```python
from build123d import *

# Parameters (mm, degrees)
SKETCH_2_R      = 3.5
EXTRUDE_3_DEPTH = 500


with BuildPart() as part:
    # Эскиз2 → Бобышка-Вытянуть3 (new body)
    with BuildSketch(Plane.XY):
        with BuildLine():
            Line((-4.25, 20.8), (4.25, 20.8))
            Line((4.25, 20.8), (8.25, 24.8))
            Line((8.25, 24.8), (8.25, 26.8))
            Line((8.25, 26.8), (4.1, 26.8))
            Line((4.1, 26.8), (4.1, 29))
            Line((4.1, 29), (9.55, 29))
            ThreePointArc((9.55, 29), (9.903553391, 29.146446609), (10.05, 29.5))
            Line((10.05, 29.5), (10.05, 30))
            Line((10.05, 30), (27.5, 30))
            ThreePointArc((27.5, 30), (29.267766953, 29.267766953), (30, 27.5))
            Line((30, 27.5), (30, 22.55))
            Line((30, 22.55), (29, 22.55))
            Line((29, 22.55), (29, 19.1))
            Line((29, 19.1), (26.8, 19.1))
            Line((26.8, 19.1), (26.8, 23.25))
            Line((26.8, 23.25), (24.8, 23.25))
            Line((24.8, 23.25), (20.8, 19.25))
            Line((20.8, 19.25), (20.8, 10.75))
            Line((20.8, 10.75), (24.8, 6.75))
            Line((24.8, 6.75), (26.8, 6.75))
            Line((26.8, 6.75), (26.8, 10.9))
            Line((26.8, 10.9), (29, 10.9))
            Line((29, 10.9), (29, 0))
            Line((29, 0), (25.8, 0))
            Line((25.8, 0), (25.8, 4.05))
            Line((25.8, 4.05), (23.398780669, 4.05))
            Line((23.398780669, 4.05), (19.248780669, 8.2))
            Line((19.248780669, 8.2), (15, 8.2))
            ThreePointArc((15, 8.2), (10.191673888, 10.191673888), (8.2, 15))
            ThreePointArc((8.2, 15), (7.965685425, 15.565685425), (7.4, 15.8))
            Line((7.4, 15.8), (-7.4, 15.8))
            ThreePointArc((-7.4, 15.8), (-7.965685425, 15.565685425), (-8.2, 15))
            ThreePointArc((-8.2, 15), (-10.191673888, 10.191673888), (-15, 8.2))
            Line((-15, 8.2), (-19.248780669, 8.2))
            Line((-19.248780669, 8.2), (-23.398780669, 4.05))
            Line((-23.398780669, 4.05), (-25.8, 4.05))
            Line((-25.8, 4.05), (-25.8, 0))
            Line((-25.8, 0), (-29, 0))
            Line((-29, 0), (-29, 10.9))
            Line((-29, 10.9), (-26.8, 10.9))
            Line((-26.8, 10.9), (-26.8, 6.75))
            Line((-26.8, 6.75), (-24.8, 6.75))
            Line((-24.8, 6.75), (-20.8, 10.75))
            Line((-20.8, 10.75), (-20.8, 19.25))
            Line((-20.8, 19.25), (-24.8, 23.25))
            Line((-24.8, 23.25), (-26.8, 23.25))
            Line((-26.8, 23.25), (-26.8, 19.1))
            Line((-26.8, 19.1), (-29, 19.1))
            Line((-29, 19.1), (-29, 22.55))
            Line((-29, 22.55), (-30, 22.55))
            Line((-30, 22.55), (-30, 27.5))
            ThreePointArc((-30, 27.5), (-29.267766953, 29.267766953), (-27.5, 30))
            Line((-27.5, 30), (-10.05, 30))
            Line((-10.05, 30), (-10.05, 29.5))
            ThreePointArc((-10.05, 29.5), (-9.903553391, 29.146446609), (-9.55, 29))
            Line((-9.55, 29), (-4.1, 29))
            Line((-4.1, 29), (-4.1, 26.8))
            Line((-4.1, 26.8), (-8.25, 26.8))
            Line((-8.25, 26.8), (-8.25, 24.8))
            Line((-8.25, 24.8), (-4.25, 20.8))
        make_face()
        with Locations((15, 15)):
            Circle(SKETCH_2_R, mode=Mode.SUBTRACT)
        with Locations(Location((-15, 15, 0), (0, 0, 180))):
            Circle(SKETCH_2_R, mode=Mode.SUBTRACT)
        with BuildLine():
            Line((14, 26.75), (19, 26.75))
            ThreePointArc((19, 26.75), (21.5, 24.25), (19, 21.75))
            Line((19, 21.75), (14, 21.75))
            ThreePointArc((14, 21.75), (11.5, 24.25), (14, 26.75))
        make_face(mode=Mode.SUBTRACT)
        with BuildLine():
            Line((-14, 21.75), (-19, 21.75))
            ThreePointArc((-19, 21.75), (-21.5, 24.25), (-19, 26.75))
            Line((-19, 26.75), (-14, 26.75))
            ThreePointArc((-14, 26.75), (-11.5, 24.25), (-14, 21.75))
        make_face(mode=Mode.SUBTRACT)
    extrude_3 = extrude(amount=EXTRUDE_3_DEPTH)

    # Зеркальное отражение13: Бобышка-Вытянуть3 across plane
    add(extrude_3.mirror(Plane(origin=(25.8, 0, 500), x_dir=(0, 0, 1), z_dir=(0, 1, 0))))


solid = part.part
```
The listing builds one solid part. Answer for the finished solid, in the listing's coordinates (mm). A direction names the side the tool comes from. Round coordinates to 2 decimals unless told otherwise and drop trailing zeros. Use one line per item in the form item = value. Start each with the question number.
1. A tool of negligible diameter and unlimited length cuts with its end or side. For faces 1 (the face through (29, 0, 246)), 2 (the face through (19, 30, 246)), 3 (the face through (-29, 0, 246)), 4 (the face through (0, -15.8, 246)), 5 (the face through (19, -30, 246)), from which of +Z, -Z, +X, -X, +Y, -Y can it reach the whole face along a straight path? Write none if from no direction.
2. Consider line 1 (Y direction, x = -15, z = 292); line 2 (X direction, y = -24, z = 233.5); line 3 (Y direction, x = -6, z = 358). Determine where each line is inside the solid, lowest interval first. Write a range as [from, to].
3. For a pull along Y with two mould halves and no side action, classify faces 6 (the face through (-19, 30, 246)), 7 (the face through (0, -20, 0)), 8 (the face through (20.8, 15, 246)), 9 (the face through (-25.8, 0, 246)) as pulls with the +Y half, pulls with the -Y half, needs draft (parallel to the pull), parting line crosses it, or undercut.
4. Given pin 1 Ø1.5 at (y, z) = (-14.5, 395) entering from -X; pin 2 Ø5 at (x, z) = (0.5, 69.5) entering from -Y; pin 3 Ø4.5 at (x, z) = (-6.5, 358) entering from +Y, each flat-ended and moving along its own axis, determine where each tip first touches the part or whether it passes through.
5. The part is cut by section A-A on z = 284. Give the number of separate pieces and of enclosed holes in the cut face, then the cut area to 3 significant figures.
Geometry check:
q1.face_1 = +Z, -Z, +X
q1.face_2 = +Z, -Z, +X, -X, +Y
q1.face_3 = +Z, -Z, -X
q1.face_4 = +Z, -Z
q1.face_5 = +Z, -Z, +X, -X, -Y
q2.line_1 = [-30, -26.75], [-21.75, -18.5], [-11.5, -8.2], [8.2, 11.5], [18.5, 21.75], [26.75, 30]
q2.line_2 = [-30, -21.49], [-11.51, -7.45], [7.45, 11.51], [21.49, 30]
q2.line_3 = [-29, -26.8], [-22.55, -15.8], [15.8, 22.55], [26.8, 29]
q3.face_6 = pulls with the +Y half
q3.face_7 = needs draft
q3.face_8 = undercut
q3.face_9 = undercut
q4.pin_1 = -20.8
q4.pin_2 = -20.8
q4.pin_3 = 29
q5.separate_pieces = 1
q5.enclosed_holes = 9
q5.area = 1,470 mm^2
